```python
from build123d import *

# Parameters (mm, degrees)
BOSS_EXTRUDE1_DEPTH              = 3.175
SKETCH7_W                        = 3.048
SKETCH7_H                        = 19.05
CUT_EXTRUDE1_DEPTH               = 3.175
FILLET1_R                        = 6.35
F_10_0_1935_DIAMETER_HOLE2_D     = 4.9149
F_10_0_1935_DIAMETER_HOLE2_DEPTH = 9.699415072
F_10_0_1935_DIAMETER_HOLE2_TIP   = 1.476584928


with BuildPart() as part:
    # Sketch1 → Boss-Extrude1 (new body)
    with BuildSketch(Plane(origin=(0, 0, 0), x_dir=(0, 0, -1), z_dir=(1, 0, 0))):
        Polygon((55.245, 0), (55.245, 36.15436), (20.9147283, 36.15436), (0, 26.034021846), (0, 0), align=None)
    extrude(amount=BOSS_EXTRUDE1_DEPTH)

    # Sketch7 → Cut-Extrude1 (cut)
    with BuildSketch(Plane.ZY):
        with Locations((-43.596153092, 23.625208274)):
            Rectangle(SKETCH7_W, SKETCH7_H)
        with Locations((-18.323153092, 20.450208274)):
            Rectangle(SKETCH7_W, SKETCH7_H)
    extrude(amount=-CUT_EXTRUDE1_DEPTH, mode=Mode.SUBTRACT)

    # Fillet1
    fillet1_edges = [part.edges().sort_by_distance(p)[0] for p in [
        (1.5875, 0, 0),
        (1.5875, 26.034021846, 0),
        (1.5875, 36.15436, -55.245),
        (1.5875, 0, -55.245),
    ]]
    fillet(fillet1_edges, radius=FILLET1_R)

    # #10 (0.1935) Diameter Hole2
    with Locations(Plane.ZY):
        with Locations((-30.896153092, 9.525), (-30.896153092, 26.67), (-7.083653092, 9.525)):
            Hole(F_10_0_1935_DIAMETER_HOLE2_D / 2, depth=F_10_0_1935_DIAMETER_HOLE2_DEPTH)
            with Locations((0, 0, -(F_10_0_1935_DIAMETER_HOLE2_DEPTH + F_10_0_1935_DIAMETER_HOLE2_TIP / 2))):  # 118° drill point
                Cone(0, F_10_0_1935_DIAMETER_HOLE2_D / 2, F_10_0_1935_DIAMETER_HOLE2_TIP, mode=Mode.SUBTRACT)


solid = part.part
```
CAD build for the part. Positions are in the model's coordinates, mm. A direction names the side the tool comes from. Coordinates: 2 decimals unless noted, no trailing zeros. Write each loop counter-clockwise with the first axis right and the second up, starting at its lowest first coordinate (ties: lowest second). Pieces come first, ordered by that corner, then holes. Notation, with made-up numbers: (-28, 31) -> (-4, 31) arc R24 ccw to (-4, 46) -> close; hole circle Ø4 at (32, 3.25). An arc over 180 degrees is marked (long way). Return JSON: item names as keys, results as strings. Group by question number.
Q1. Which spindle directions (+Z, -Z, +X, -X, +Y, -Y) get a long thin tool onto all of the face, cutting with end or side? Do faces 5 (the face through (1.57, 32.02, -12.37)), 6 (the face through (2, 20, -16.799)). Say none if no direction does.
Q2. Cut at B-B, the plane z = -5.5. Give the cut face in (x, y) (3 decimals).
Q3. Cut at D-D, the plane z = -30. Give the cut face in (x, y) (3 decimals), then the cut area to 3 significant figures.
Q4. Drill centre lines: line 1 (Z direction, x = 0.75, y = 17.5) (3 decimals); line 2 (Y direction, x = 1.8, z = -43); line 3 (Z direction, x = 1.85, y = 6). Where is each one in solid material? Low to high.
Q5. Flat gauge pins, fed straight in: pin 1 (4 mm diameter, centred on y = 26.67, z = -30.9, fed in from +X); pin 2 (8 mm diameter, centred on y = 9.52, z = -30.9, fed in from +X) (3 decimals); pin 3 (1 mm diameter, centred on x = 0.5, y = 30.5, fed in from -Z). Where does each tip first touch, or does it go through?
Q6. Pull direction Z, two halves, no side cores. Call faces 1 (the face through (1.61, 1.81, -1.91)), 2 (the face through (2, 29.975, -18)), 3 (the face through (0, 18, -27)), 4 (the face through (2, 33.15, -44)): released by +Z, released by -Z, zero draft, split by the parting line, or undercut.
Q7. Cut at A-A, the plane y = 26.67. Give the cut face in (x, z) (3 decimals).
Q8. Cut at C-C, the plane x = 1.8. Give the cut face in (y, z) (3 decimals), then the cut area to 3 significant figures.
Returned:
{
 "1": {"face 5": "+Z, +X, -X, +Y", "face 6": "+X, -X"},
 "2": {"outline": "(0, 0.057) -> (3.175, 0.057) -> (3.175, 7.646) -> (0, 7.646) -> close; (0, 11.404) -> (3.175, 11.404) -> (3.175, 28.695) -> (0, 28.695) -> close"},
 "3": {"outline": "(0, 0) -> (3.175, 0) -> (3.175, 7.237) -> (0, 7.237) -> close; (0, 11.813) -> (3.175, 11.813) -> (3.175, 24.382) -> (0, 24.382) -> close; (0, 28.958) -> (3.175, 28.958) -> (3.175, 36.154) -> (0, 36.154) -> close", "area": "85.7 mm2"},
 "4": {"line 1": "z = -55.245 to -45.12, -42.072 to -19.847, -16.799 to 0", "line 2": "y = 0 to 14.1, 33.15 to 36.15", "line 3": "z = -55.24 to -0.01"},
 "5": {"pin 1": "passes through", "pin 2": "stops at x = 3.175", "pin 3": "stops at z = -55.24"},
 "6": {"face 1": "released by +Z", "face 2": "undercut", "face 3": "zero draft", "face 4": "undercut"},
 "7": {"outline": "(0, -55.245) -> (3.175, -55.245) -> (3.175, -45.12) -> (0, -45.12) -> close; (0, -42.072) -> (3.175, -42.072) -> (3.175, -33.354) -> (0, -33.354) -> close; (0, -28.439) -> (3.175, -28.439) -> (3.175, -19.847) -> (0, -19.847) -> close; (0, -16.799) -> (3.175, -16.799) -> (3.175, -1.991) -> (0, -1.991) -> close"},
 "8": {"outline": "(0, -48.895) arc R6.35 ccw to (6.35, -55.245) -> (29.804, -55.245) arc R6.35 ccw to (36.154, -48.895) -> (36.154, -20.915) -> (27.768, -3.584) arc R6.35 ccw to (22.052, 0) -> (6.35, 0) arc R6.35 ccw to (0, -6.35) -> close; hole circle Ø4.915 at (9.525, -30.896); hole circle Ø4.915 at (9.525, -7.084); hole (10.925, -19.847) -> (29.975, -19.847) -> (29.975, -16.799) -> (10.925, -16.799) -> close; hole (14.1, -45.12) -> (33.15, -45.12) -> (33.15, -42.072) -> (14.1, -42.072) -> close; hole circle Ø4.915 at (26.67, -30.896)", "area": "1,690 mm2"}
}
